Can you work these out from the model? Positions are in its coordinate system, mm. Give positions to 0.01 mm unless a question says otherwise; leave off trailing zeros. Loops run counter-clockwise (first coordinate to the right, second up) from the corner with the lowest first, then second, coordinate; pieces in that order, holes last. Notation, with made-up numbers: (48, -10) - (105, -10) arc R27 ccw to (105, 10) - close; hole circle Ø3 at (53, 13). An arc over 180 degrees is marked (long way). Write item = value, one per line.
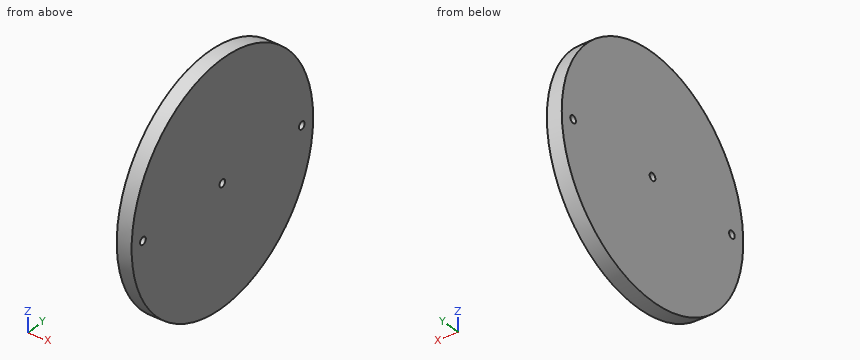
from build123d import *

# Parameters (mm, degrees)
F0_R     = 101.6
F2_DEPTH = 12.7
F3_D     = 6.35
F5_D     = 6.35
F7_D     = 6.35


with BuildPart() as f2:
    # F0 (on Right) → F2 (new body)
    with BuildSketch(Plane.YZ):
        Circle(F0_R)
    extrude(amount=F2_DEPTH)

    # F3 (through all)
    with Locations(Plane(origin=(0, 0, 0), x_dir=(0, 1, 0), z_dir=(-1, 0, 0))):
        with Locations((0, 0)):
            Hole(F3_D / 2)

    # F5 (through all)
    with Locations(Plane.YZ.offset(12.7)):
        with Locations((88.9, 0)):
            Hole(F5_D / 2)

    # F7 (through all)
    with Locations(Plane.YZ.offset(12.7)):
        with Locations((-88.9, 0)):
            Hole(F7_D / 2)


solid = f2.part
Q1. I need wall thicknesses on L1, parallel to Z at x = 9.75, y = 0 (3 decimals); L2, parallel to Z at x = 8.5, y = -88.9 (3 decimals); L3, parallel to Z at x = 6, y = 22.5. Which ranges of each line are inside material? Lowest first, please.
Output:
L1 = -101.6 to -3.175, 3.175 to 101.6
L2 = -49.187 to -3.175, 3.175 to 49.187
L3 = -99.08 to 99.08
Q2. Imagine slicing it at A-A, the plane z = 0. Write out the boundary of the cut face in (x, y) (3 decimals).
Output:
outline = (0, -101.6) - (12.7, -101.6) - (12.7, -92.075) - (0, -92.075) - close; (0, -85.725) - (12.7, -85.725) - (12.7, -3.175) - (0, -3.175) - close; (0, 3.175) - (12.7, 3.175) - (12.7, 85.725) - (0, 85.725) - close; (0, 92.075) - (12.7, 92.075) - (12.7, 101.6) - (0, 101.6) - close
Q3. Imagine slicing it at D-D, the plane z = 22. Write out the boundary of the cut face in (x, y), then the cut area to 3 significant figures.
Output:
outline = (0, -99.19) - (12.7, -99.19) - (12.7, 99.19) - (0, 99.19) - close
area = 2,520 mm2
Q4. Imagine slicing it at B-B, the plane y = -88.9. Write out the boundary of the cut face in (x, z) (3 decimals), then the cut area to 3 significant figures.
Output:
outline = (0, -49.187) - (12.7, -49.187) - (12.7, -3.175) - (0, -3.175) - close; (0, 3.175) - (12.7, 3.175) - (12.7, 49.187) - (0, 49.187) - close
area = 1,170 mm2
Q5. For pin 1 (4 mm diameter, centred on x = 8.5, y = 68.5, fed in from -Z); pin 2 (6 mm diameter, centred on x = 6, z = 41, fed in from +Y); pin 3 (5 mm diameter, centred on x = 3, z = 71, fed in from -Y), each with a flat end and sliding along its axis, tell me the tip position at first contact or that it passes through.
Output:
pin_1 = -76.81
pin_2 = 94.23
pin_3 = -75.04
Q6. Imagine slicing it at C-C, the plane x = 3.25. Write out the boundary of the cut face in (y, z) (3 decimals), then the cut area to 3 significant figures.
Output:
outline = circle Ø203.2 at (0, 0); hole circle Ø6.35 at (-88.9, 0); hole circle Ø6.35 at (0, 0); hole circle Ø6.35 at (88.9, 0)
area = 32,300 mm2
